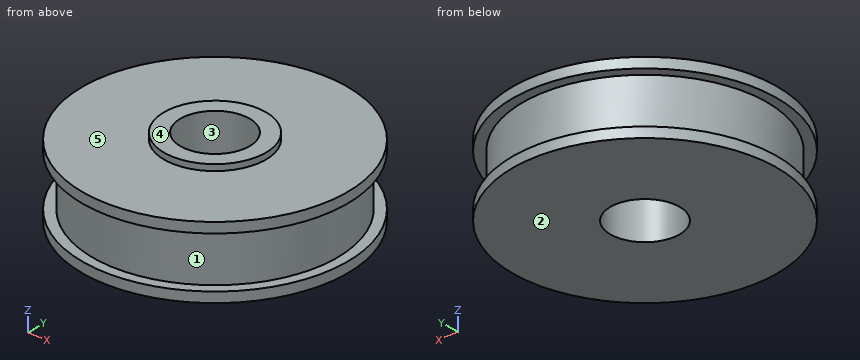
from build123d import *

# Parameters (mm, degrees)
SKETCH1_R           = 6.5
BOSS_EXTRUDE1_DEPTH = 3.5
SKETCH2_R           = 2.5
BOSS_EXTRUDE2_DEPTH = 0.3
SKETCH3_R           = 6.5
SKETCH3_R_2         = 6
CUT_EXTRUDE1_DEPTH  = 2.5
SKETCH4_R           = 1.7
CUT_EXTRUDE2_DEPTH  = 4.8


with BuildPart() as part:
    # Sketch1 → Boss-Extrude1 (new body)
    with BuildSketch(Plane.XY):
        Circle(SKETCH1_R)
    extrude(amount=BOSS_EXTRUDE1_DEPTH)

    # Sketch2 → Boss-Extrude2 (add)
    with BuildSketch(Plane.XY.offset(3.5)):
        Circle(SKETCH2_R)
    extrude(amount=BOSS_EXTRUDE2_DEPTH)

    # Sketch3 → Cut-Extrude1 (cut)
    with BuildSketch(Plane(origin=(0, 0, 0.5), x_dir=(-1, 0, 0), z_dir=(0, 0, -1))):
        Circle(SKETCH3_R)
        Circle(SKETCH3_R_2, mode=Mode.SUBTRACT)
    extrude(amount=-CUT_EXTRUDE1_DEPTH, mode=Mode.SUBTRACT)

    # Sketch4 → Cut-Extrude2 (cut, through all)
    with BuildSketch(Plane.XY.offset(3.8)):
        Circle(SKETCH4_R)
    extrude(amount=-CUT_EXTRUDE2_DEPTH, mode=Mode.SUBTRACT)


solid = part.part
Input: part model. Units: mm. Frame: model coordinates. Face numbers are marked on the shaded views. A direction names the side the tool comes from. Coordinates: 2 decimals unless noted, no trailing zeros. Write each loop counter-clockwise with the first axis right and the second up, starting at its lowest first coordinate (ties: lowest second). Pieces come first, ordered by that corner, then holes. Notation, with made-up numbers: M -31.75,-32.75 L -6.75,-32.75 A15 cw -6.75,-23.75 Z; hole C 57,17 d3. An arc over 180 degrees is marked long. Answer as a JSON object with one key per item and string values. Group by question number.
(1) Ray query, line 1 along Y through (x, z) = (0, 1.9); line 2 along Z through (x, y) = (-4.75, -1.5); line 3 along X through (y, z) = (-1, 3.25). Return the intervals inside material, ascending. Write a range as [from, to].
(2) Section D-D on y = -4.25. Output: boundary loops of the cut face in (x, z).
(3) Mould query, pull axis Y, two halves, no side actions, for the marked faces 1, 2 and 3. Classes: pulls with the +Y half, pulls with the -Y half, needs draft (parallel to the pull), parting line crosses it, or undercut.
(4) Section A-A on y = 0. Output: boundary loops of the cut face in (x, z).
(5) Section C-C on z = 0.3. Output: boundary loops of the cut face in (x, y), plus the area to 3 significant figures.
(6) Contact query for flat-ended pins moving along their axis: P1, Ø6.5, axis at x = -3, y = 2.5, coming from the +Z side; P2, Ø2, axis at x = 1, z = 2.5, coming from the -Y side; P3, Ø1.5, axis at x = 0.5, z = 1.5, coming from the -Y side. Output: stop coordinate, or through.
(7) Set-up query: the marked faces 4 and 5. Return all of +Z, -Z, +X, -X, +Y, -Y with unobstructed straight access to the full face (end or side cutting, diameter ignored); none if empty.
Result set:
{
 "1": {"line 1": "y = [-6, -1.7], [1.7, 6]", "line 2": "z = [0, 3.5]", "line 3": "x = [-6.42, -1.37], [1.37, 6.42]"},
 "2": {"outline": "M -4.92,0 L 4.92,0 L 4.92,0.5 L 4.24,0.5 L 4.24,3 L 4.92,3 L 4.92,3.5 L -4.92,3.5 L -4.92,3 L -4.24,3 L -4.24,0.5 L -4.92,0.5 Z"},
 "3": {"face 1": "parting line crosses it", "face 2": "needs draft", "face 3": "undercut"},
 "4": {"outline": "M -6.5,0 L -1.7,0 L -1.7,3.8 L -2.5,3.8 L -2.5,3.5 L -6.5,3.5 L -6.5,3 L -6,3 L -6,0.5 L -6.5,0.5 Z; M 1.7,0 L 6.5,0 L 6.5,0.5 L 6,0.5 L 6,3 L 6.5,3 L 6.5,3.5 L 2.5,3.5 L 2.5,3.8 L 1.7,3.8 Z"},
 "5": {"outline": "C 0,0 d13; hole C 0,0 d3.4", "area": "124 mm2"},
 "6": {"P1": "stops at z = 3.8", "P2": "stops at y = -6.5", "P3": "stops at y = -6"},
 "7": {"face 4": "+Z, +X, -X, +Y, -Y", "face 5": "+Z"}
}
